from build123d import *

# Parameters (mm, degrees)
F1_DEPTH = 12.7
F2_R     = 50.8
F3_R     = 25.4


with BuildPart() as f1:
    # F0 (on Top) → F1 (new body)
    with BuildSketch(Plane.XY):
        Polygon((-50.8, 381), (-127, 381), (-127, 0), (-127, -381), (-50.8, -381), (-50.8, -533.4), (50.8, -533.4), (50.8, -381), (127, -381), (127, 0), (127, 381), (50.8, 381), (50.8, 533.4), (-50.8, 533.4), align=None)
    extrude(amount=F1_DEPTH)

    # F2
    f2_edges = [f1.edges().sort_by_distance(p)[0] for p in [
        (-50.8, 381, 6.35),
        (50.8, 381, 6.35),
        (-50.8, -381, 6.35),
        (50.8, -381, 6.35),
    ]]
    fillet(f2_edges, radius=F2_R)

    # F3
    f3_edges = [f1.edges().sort_by_distance(p)[0] for p in [
        (-50.8, -533.4, 6.35),
        (50.8, -533.4, 6.35),
        (50.8, 533.4, 6.35),
        (-50.8, 533.4, 6.35),
    ]]
    fillet(f3_edges, radius=F3_R)


solid = f1.part
Input: part model. Units: mm. Frame: model coordinates. Round coordinates to 2 decimals unless told otherwise and drop trailing zeros. Write each loop counter-clockwise with the first axis right and the second up, starting at its lowest first coordinate (ties: lowest second). Pieces come first, ordered by that corner, then holes.
1) Contact query for flat-ended pins moving along their axis: P1, Ø4, axis at x = -112, z = 3.5, coming from the -Y side; P2, Ø2, axis at y = -405, z = 2, coming from the -X side; P3, Ø4, axis at y = 459, z = 4, coming from the -X side. Output: stop coordinate, or through.
2) Cut plane C-C (x = 67). Return the cut outline in (y, z), then the cut area to 3 significant figures.
3) Cut plane B-B (y = -458.5). Return the cut outline in (x, z), then the cut area to 3 significant figures.
4) Ray query, L1, parallel to X at y = 486, z = 1.5; L2, parallel to Y at x = -28.5, z = 0.5; L3, parallel to Y at x = -98.5, z = 1.5. Return the intervals inside material, ascending.
5) Cut plane A-A (z = 10). Return the cut outline in (x, y), then the cut area to 3 significant figures.
Geometry says:
1. P1: stops at y = -381
1. P2: stops at x = -59.08
1. P3: stops at x = -50.8
2. outline: (-394.6, 0) - (394.6, 0) - (394.6, 12.7) - (-394.6, 12.7) - close
2. area: 10,000 mm2
3. outline: (-50.8, 0) - (50.8, 0) - (50.8, 12.7) - (-50.8, 12.7) - close
3. area: 1,290 mm2
4. L1: x = -50.8 to 50.8
4. L2: y = -533.21 to 533.21
4. L3: y = -381.09 to 381.09
5. outline: (-127, -381) - (-101.6, -381) arc R50.8 cw to (-50.8, -431.8) - (-50.8, -508) arc R25.4 ccw to (-25.4, -533.4) - (25.4, -533.4) arc R25.4 ccw to (50.8, -508) - (50.8, -431.8) arc R50.8 cw to (101.6, -381) - (127, -381) - (127, 381) - (101.6, 381) arc R50.8 cw to (50.8, 431.8) - (50.8, 508) arc R25.4 ccw to (25.4, 533.4) - (-25.4, 533.4) arc R25.4 ccw to (-50.8, 508) - (-50.8, 431.8) arc R50.8 cw to (-101.6, 381) - (-127, 381) - close
5. area: 226,000 mm2
